Verification items for the finished model (mm, model axes). Face numbers are marked on the shaded views. Coordinates: 2 decimals unless noted, no trailing zeros. Order: outer loops, then holes, each group sorted by start corner. A loop starts at its lowest first (then second) coordinate and runs counter-clockwise, first axis right, second up. Notation, with made-up numbers: M 38.5,-30.75 L 76.5,-30.75 A11 ccw 76.5,-12.75 Z; hole C -35,75.5 d8. An arc over 180 degrees is marked long. Return JSON: item names as keys, results as strings. Group by question number.
Q1. Thickness scan on probe 1 along X at (y, z) = (14.2, 0.75) (3 decimals); probe 2 along Z at (x, y) = (13, 0.25); probe 3 along Y at (x, z) = (39.8, 4) (3 decimals). Record the ranges inside material, lowest first.
Q2. Section check C-C, the plane y = 13.5. Enter the section's corners in (x, z), then the cut area to 3 significant figures.
Q3. Section check A-A, the plane z = 9.5. Enter the section's corners in (x, y) (3 decimals), then the cut area to 3 significant figures.
Q4. Mould release check, pull along Z, two halves, no side actions. Record for the marked faces 1, 2, 3 and 4: pulls with the +Z half, pulls with the -Z half, needs draft (parallel to the pull), parting line crosses it, or undercut.
Q5. Section check D-D, the plane x = 39.8. Enter the section's corners in (y, z) (3 decimals), then the cut area to 3 significant figures.
Q6. Go/stop test with flat-tipped pins: pin 1 Ø7 at (x, y) = (40.5, 13) entering from +Z; pin 2 Ø5.5 at (x, y) = (39.8, 14.2) entering from -Z; pin 3 Ø3 at (x, y) = (3, 8.5) entering from -Z; pin 4 Ø3 at (x, y) = (39.8, 14.2) entering from +Z. Record where each tip stops, or that it passes through.
Q7. Section check B-B, the plane x = 31. Enter the section's corners in (y, z), then the cut area to 3 significant figures.
Autodesk Inventor part; units mm, degrees
ref_plane "YZ Plane" through (0, 0, 0) normal (1, 0, 0) x (0, 1, 0)
ref_plane "XZ Plane" through (0, 0, 0) normal (0, 1, 0) x (-1, 0, 0)
ref_plane "XY Plane" through (0, 0, 0) normal (0, 0, 1) x (1, 0, 0)
sketch "Sketch1" plane through (0, 0, 0) normal (0, 1, 0) x (-1, 0, 0)
  line L0 (-25, 12.5) -> (25, 12.5)
  line L1 (25, 12.5) -> (25, -12.5)
  line L2 (25, -12.5) -> (-25, -12.5)
  line L3 (-25, -12.5) -> (-25, 12.5)
  line L4 (-25, 12.5) -> (25, -12.5) construction
  line L5 (25, 12.5) -> (-25, -12.5) construction
  line L6 (27, 14) -> (27, -14)
  line L7 (-25, 12.5) -> (-25, 14)
  line L8 (-25, 14) -> (27, 14)
  line L9 (27, -14) -> (-25, -14)
  line L10 (-25, -14) -> (-25, -12.5)
  line L11 (25, 12.5) -> (27, 12.5)
  line L12 (25, -12.5) -> (27, -12.5)
  line L13 (-25, -14) -> (27, -14)
  line L14 (27, -14) -> (27, -22)
  line L15 (27, -22) -> (-25, -22)
  line L16 (-25, -22) -> (-25, -14)
  line L17 (27, 0) -> (-25, 0)
  line L18 (-25, 14) -> (27, 14)
  line L19 (27, 14) -> (27, 22)
  line L20 (27, 22) -> (-25, 22)
  line L21 (-25, 22) -> (-25, 14)
  point P0 (0, 0)
  point P1 (27, 14)
  dimension "d0" = 25
  dimension "d1" = 50
  dimension "d2" = 2
  dimension "d3" = 1.5
  dimension "d4" = 1.5
  dimension "d60" = 8
extrude "Extrusion1" add sketch "Sketch1" against normal blind 2 contours L7 L8 L6 L11 L0 | L0 L1 L17 L3 | L11 L6 L17 L1 | L17 L1 L2 L3 | L17 L6 L12 L1 | L2 L12 L6 L9 L10
extrude "Extrusion2" add sketch "Sketch1" along normal blind 18.8 contours L7 L8 L6 L11 L0 | L2 L12 L6 L9 L10
sketch "Sketch2" plane through (-27, 0, -12.5) normal (0, 0, 1) x (1, 0, 0)
  line L0 (0, 18.8) -> (0, 20)
  line L1 (0, 0) -> (0, 18.8)
  line L2 (0, 18.8) -> (2, 18.8)
  line L3 (0, 18.8) -> (52, 18.8)
  line L4 (2, 18.8) -> (2, 11.5)
  line L5 (52, 0) -> (0, 0)
  line L6 (2, 11.5) -> (0, 11.5)
  line L7 (0, -2) -> (0, 18.8)
  point P0 (27, 0)
  dimension "d13" = 11.5
  dimension "d14" = 20
  dimension "d15" = 2
extrude "Extrusion3" add sketch "Sketch2" along normal up to surface (25 mm away)
sketch "Sketch4" plane through (-27, -2, 14) normal (0, 0, 1) x (1, 0, 0)
  circle A0 centre (66.8, 16.2) radius 2.575
  circle A1 centre (66.8, 16.2) radius 3.1
  circle A2 centre (66.8, 16.2) radius 3.8
  line L0 (52, 2) -> (52, 20.8)
  line L1 (52, 12) -> (70.6, 12)
  line L2 (70.6, 12) -> (70.6, 20.8)
  line L3 (70.6, 20.8) -> (52, 20.8)
  point P0 (27, 2)
  dimension "d31" = 5.15
  dimension "d32" = 6.2
  dimension "d33" = 0.7
  dimension "d34" = 10
  dimension "d35" = 14.2
  dimension "d61" = 18.6
extrude "Extrusion4" add sketch "Sketch4" against normal up to surface (28 mm away) contours A1 | A2 | L2 L1 L0 L3
sketch "Sketch5" plane through (25, -2, 14) normal (1, 0, 0) x (0, 0, -1)
  line L0 (0, 0) -> (0, 12)
  line L1 (0, 2) -> (28, 2)
  line L2 (28, 0) -> (28, 12)
  line L3 (1.5, 2) -> (26.5, 2)
  line L4 (28, 12) -> (26.5, 12)
  line L5 (26.5, 2) -> (26.5, 12)
  line L6 (1.5, 12) -> (1.5, 2)
  line L7 (26.5, 12) -> (1.5, 12)
  line L8 (26.5, 12) -> (26.5, 20.8)
  line L9 (26.5, 20.8) -> (28, 20.8)
  line L10 (28, 20.8) -> (28, 12)
  line L11 (28, 12) -> (28, 0)
  line L12 (28, 0) -> (0, 0)
  line L13 (0, 0) -> (0, 12)
  line L14 (0, 12) -> (0, 20.8)
  line L15 (0, 20.8) -> (1.5, 20.8)
  line L16 (1.5, 20.8) -> (1.5, 12)
  line L17 (1.5, 12) -> (0, 12)
  line L18 (1.5, 20.8) -> (26.5, 20.8)
  line L19 (1.5, 2) -> (26.5, 2)
  point P0 (14, 2)
extrude "Extrusion6" add sketch "Sketch5" along normal up to surface (18.6 mm away) contours L0 L1 L2 L12
extrude "Extrusion8" add sketch "Sketch5" along normal blind 4 contours L0 L17 L6 L1 | L1 L5 L4 L2
extrude "Extrusion9" add sketch "Sketch4" along normal blind 1 contours A2
extrude "Extrusion10" add sketch "Sketch4" along normal blind 0.1 contours A1
sketch "Sketch7" plane through (-27, -2, -14) normal (0, 0, -1) x (-1, 0, 0)
  circle A0 centre (-66.8, 16.2) radius 3.8
  circle A1 centre (-66.8, 16.2) radius 3.1
  circle A2 centre (-66.8, 16.2) radius 3.1
  circle A3 centre (-66.8, 16.2) radius 2.575
  point P0 (-27, 2)
extrude "Extrusion11" add sketch "Sketch7" along normal blind 0.1 contours A1
extrude "Extrusion12" add sketch "Sketch7" along normal blind 1 contours A0
extrude "Extrusion13" add sketch "Sketch1" against normal up to surface (2 mm away) contours L21 L20 L19 L8 | L9 L14 L15 L16
sketch "Sketch8" plane through (25, 0, 22) normal (1, 0, 0) x (0, 0, -1)
  line L0 (0, -2) -> (8, -2)
  line L1 (8, 0) -> (8, -2)
  line L2 (0, 0) -> (8, 0)
  line L3 (0, 0) -> (0, -2)
  line L4 (36, -2) -> (44, -2)
  line L5 (44, 0) -> (44, -2)
  line L6 (36, 0) -> (44, 0)
  line L7 (36, -2) -> (36, 0)
  point P0 (22, 0)
extrude "Extrusion14" add sketch "Sketch8" along normal up to surface (18.6 mm away)
equation "\"d4\" = d3"
equation "\"d15\" = d2"
properties part number "chaimber"
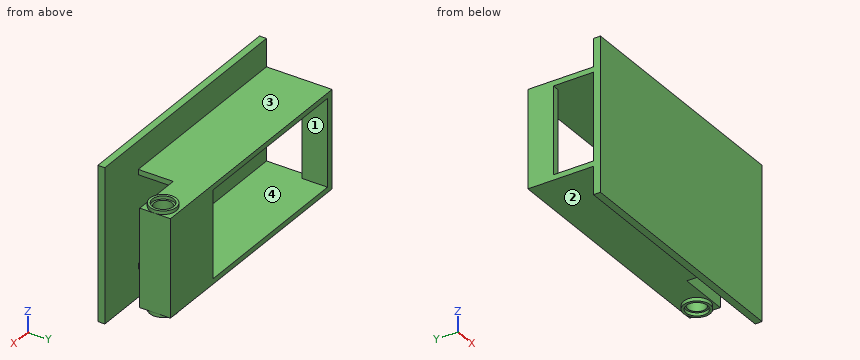
Numbers:
{
 "1": {"probe 1": "x = -27 to -25, 25 to 37.225, 42.375 to 43.6", "probe 2": "z = -14 to -12.5, 12.5 to 14", "probe 3": "y = -2 to 0, 10 to 11.625, 16.775 to 18.8"},
 "2": {"outline": "M -27,-14 L 36.07,-14 L 36.07,-15 L 36.78,-15 L 36.78,-14.1 L 37.32,-14.1 L 37.32,14.1 L 36.78,14.1 L 36.78,15 L 36.07,15 L 36.07,14 L -27,14 Z; M 42.28,-14.1 L 42.82,-14.1 L 42.82,-15 L 43.53,-15 L 43.53,-14 L 43.6,-14 L 43.6,14 L 43.53,14 L 43.53,15 L 42.82,15 L 42.82,14.1 L 42.28,14.1 Z; hole M -25,-12.5 L 25,-12.5 L 25,12.5 L -25,12.5 Z", "area": "591 mm2"},
 "3": {"outline": "M -27,-2 L 43.6,-2 L 43.6,0 L -27,0 Z; M -27,11.5 L -25,11.5 L -25,18.8 L -27,18.8 Z; M 25,10 L 43.6,10 L 43.6,18.8 L 25,18.8 Z; hole C 39.8,14.2 d5.15", "area": "299 mm2"},
 "4": {"face 1": "undercut", "face 2": "pulls with the -Z half", "face 3": "pulls with the +Z half", "face 4": "undercut"},
 "5": {"outline": "M -2,-22 L 0,-22 L 0,22 L -2,22 Z; M 10,-14 L 10.4,-14 L 10.4,-15 L 11.1,-15 L 11.1,-14.1 L 11.625,-14.1 L 11.625,14.1 L 11.1,14.1 L 11.1,15 L 10.4,15 L 10.4,14 L 10,14 Z; M 16.775,-14.1 L 17.3,-14.1 L 17.3,-15 L 18,-15 L 18,-14 L 18.8,-14 L 18.8,14 L 18,14 L 18,15 L 17.3,15 L 17.3,14.1 L 16.775,14.1 Z", "area": "193 mm2"},
 "6": {"pin 1": "stops at z = 15", "pin 2": "stops at z = -14.1", "pin 3": "stops at z = -14", "pin 4": "passes through"},
 "7": {"outline": "M -2,-22 L 0,-22 L 0,22 L -2,22 Z; M 10,-14 L 18.8,-14 L 18.8,14 L 10,14 Z", "area": "334 mm2"}
}
